Autodesk Inventor part; units mm, degrees
ref_plane "YZ Plane" through (0, 0, 0) normal (1, 0, 0) x (0, 1, 0)
ref_plane "XZ Plane" through (0, 0, 0) normal (0, 1, 0) x (-1, 0, 0)
ref_plane "XY Plane" through (0, 0, 0) normal (0, 0, 1) x (1, 0, 0)
sketch "Szkic1" plane through (0, 0, 0) normal (0, 1, 0) x (-1, 0, 0)
  circle A0 centre (0, 0) radius 5
  circle A1 centre (0, 0) radius 3.5
  line L0 (2.4, 1.05) -> (-2.4, 1.05)
  line L1 (-2.4, 1.05) -> (-2.4, -1.05)
  line L2 (-2.4, -1.05) -> (2.4, -1.05)
  line L3 (2.4, -1.05) -> (2.4, 1.05)
  line L4 (1.05, 2.4) -> (-1.05, 2.4)
  line L5 (-1.05, 2.4) -> (-1.05, -2.4)
  line L6 (-1.05, -2.4) -> (1.05, -2.4)
  line L7 (1.05, -2.4) -> (1.05, 2.4)
  point P0 (-1.05, 0)
  point P1 (0, -1.05)
  point P2 (0, 2.4)
  point P3 (2.4, 0)
  point P4 (-1.05, 1.05)
  point P5 (1.05, 1.05)
  point P6 (1.05, -1.05)
  point P7 (-1.05, -1.05)
  dimension "d0" = 10
  dimension "d1" = 7
  dimension "d2" = 4.8
  dimension "d3" = 4.8
  dimension "d4" = 2.1
  dimension "d5" = 2.1
extrude "Wyciągnięcie proste1" add sketch "Szkic1" along normal blind 1 contours A0
extrude "Wyciągnięcie proste2" add sketch "Szkic1" along normal blind 5 contours A1
equation "\"d3\" = d2"
equation "\"d5\" = d4"
properties part number "lego1"
The model under review builds one solid part; all positions refer to its coordinate system, in mm. A direction names the side the tool comes from. Round coordinates to 2 decimals unless told otherwise and drop trailing zeros. Write each loop counter-clockwise with the first axis right and the second up, starting at its lowest first coordinate (ties: lowest second). Pieces come first, ordered by that corner, then holes. Notation, with made-up numbers: M -38.5,57 L -2.5,57 A16 ccw -2.5,84 Z; hole C -30.75,33 d9. An arc over 180 degrees is marked long. Answer as CSV lines item,"result". Start each with the question number.
Q1. Consider section B-B, the plane z = 0. Give the boundary of the cut face in (x, y).
Q2. Clearance check with flat-ended pins moving along their axes: P1, Ø1.5, axis at x = 1.5, y = 2.5, coming from the +Z side; P2, Ø1.7, axis at y = 2, z = 0.5, coming from the +X side; P3, Ø0.6, axis at x = -0.5, y = 1.5, coming from the -Z side. State where each tip first meets the part, or that it passes through.
Q3. Consider section A-A, the plane x = 0. Give the boundary of the cut face in (y, z), then the cut area to 3 significant figures.
Q4. Tool access review of faces 4 (the face through (-2, 2, -1.05)), 5 (the face through (-2.2, 1, -3.3)), 6 (the face through (-2, 0, -2)): name each direction out of +Z, -Z, +X, -X, +Y, -Y from which nothing blocks a thin tool from reaching the whole face with its end or side.
Q5. The part is to be moulded in two halves that separate along X. For faces 1 (the face through (2.4, 2, 0)), 2 (the face through (-2, 5, -2)), 3 (the face through (-3.233, 2.972, 1.341)), say which applies: +X half, -X half, draft (parallel to the pull), parting line (faces both ways), or undercut.
Q6. Consider section C-C, the plane y = 3.9. Give the boundary of the cut face in (x, z).
Q7. Wall thickness on line 1 along Z through (x, y) = (-1.5, 2.5); line 2 along Y through (x, z) = (-3.5, 2.5); line 3 along X through (y, z) = (3.3, -1.75): over which ranges is each line inside the solid? List them lowest first.
Result set:
1,outline,"M -5,0 L -2.4,0 L -2.4,5 L -3.5,5 L -3.5,1 L -5,1 Z; M 2.4,0 L 5,0 L 5,1 L 3.5,1 L 3.5,5 L 2.4,5 Z"
2,P1,"stops at z = 3.42"
2,P2,"stops at x = 3.5"
2,P3,"stops at z = -3.49"
3,outline,"M 0,-5 L 1,-5 L 1,-3.5 L 5,-3.5 L 5,-2.4 L 0,-2.4 Z; M 0,2.4 L 5,2.4 L 5,3.5 L 1,3.5 L 1,5 L 0,5 Z"
3,area,"14.0 mm²"
4,face 4,"+Y, -Y"
4,face 5,"+Y"
4,face 6,"+Z, -Z, +X, -X, -Y"
5,face 1,"undercut"
5,face 2,"draft"
5,face 3,"parting line"
6,outline,"C 0,0 d7; hole M -2.4,-1.05 L -1.05,-1.05 L -1.05,-2.4 L 1.05,-2.4 L 1.05,-1.05 L 2.4,-1.05 L 2.4,1.05 L 1.05,1.05 L 1.05,2.4 L -1.05,2.4 L -1.05,1.05 L -2.4,1.05 Z"
7,line 1,"z = -3.16 to -1.05, 1.05 to 3.16"
7,line 2,"y = 0 to 1"
7,line 3,"x = -3.03 to -1.05, 1.05 to 3.03"
